Print and shaded views of the part. All mm, measured from the part's lowest x, y and z. Round coordinates to 2 decimals unless told otherwise and drop trailing zeros. Loops run counter-clockwise (first coordinate to the right, second up) from the corner with the lowest first, then second, coordinate; pieces in that order, holes last. Notation, with made-up numbers: (41.5, 31.5) -> (85.5, 31.5) arc R18 cw to (85.5, 47.5) -> close; hole circle Ø6 at (72.5, 72.25). An arc over 180 degrees is marked (long way). Answer as CSV lines item,"result".
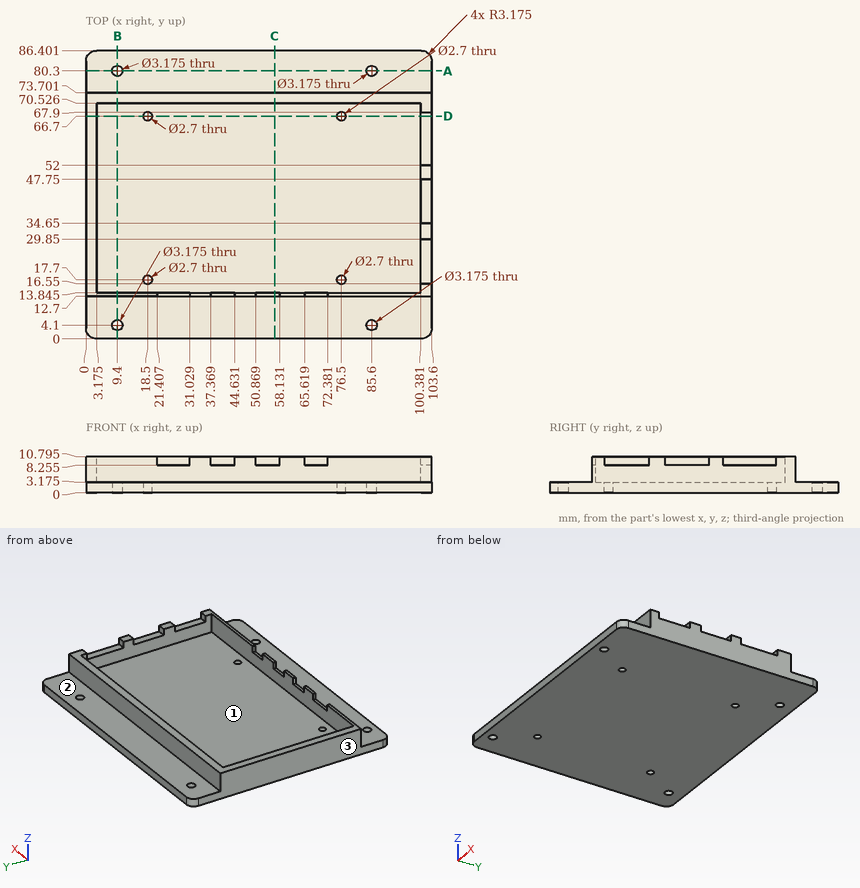
Q1. Slice it at B-B, the plane x = 9.4. Give the cut face in (y, z) (1 decimal), and give its area (3 significant figures).
Results:
outline,"(0, 0) -> (2.5, 0) -> (2.5, 3.2) -> (0, 3.2) -> close; (5.7, 0) -> (78.7, 0) -> (78.7, 3.2) -> (73.7, 3.2) -> (73.7, 10.8) -> (70.5, 10.8) -> (70.5, 3.2) -> (13.8, 3.2) -> (13.8, 10.8) -> (12.7, 10.8) -> (12.7, 3.2) -> (5.7, 3.2) -> close; (81.9, 0) -> (86.4, 0) -> (86.4, 3.2) -> (81.9, 3.2) -> close"
area,"287 mm2"
Q2. Slice it at D-D, the plane y = 66.7. Count the separate pieces of the cut face and the enclosed holes in it, and give its area (3 significant figures).
Results:
separate pieces,"3"
enclosed holes,"0"
area,"352 mm2"
Q3. Slice it at A-A, the plane y = 80.3. Give the cut face in (x, z) (1 decimal), and give its area (3 significant figures).
Results:
outline,"(0, 0) -> (7.8, 0) -> (7.8, 3.2) -> (0, 3.2) -> close; (11, 0) -> (84, 0) -> (84, 3.2) -> (11, 3.2) -> close; (87.2, 0) -> (103.6, 0) -> (103.6, 3.2) -> (87.2, 3.2) -> close"
area,"309 mm2"
Q4. Two-plate mould, pull along X, no slides. Class the marked faces 1, 2 and 3: pulls with the +X half, pulls with the -X half, needs draft (parallel to the pull), parting line crosses it, or undercut.
Results:
face 1,"undercut"
face 2,"needs draft"
face 3,"pulls with the -X half"
Q5. Slice it at C-C, the plane x = 56.5. Give the cut face in (y, z) (1 decimal), and give its area (3 significant figures).
Results:
outline,"(0, 0) -> (86.4, 0) -> (86.4, 3.2) -> (73.7, 3.2) -> (73.7, 10.8) -> (70.5, 10.8) -> (70.5, 3.2) -> (13.8, 3.2) -> (13.8, 8.3) -> (12.7, 8.3) -> (12.7, 3.2) -> (0, 3.2) -> close"
area,"304 mm2"
Q6. Drop flat-ended pins along their axis: pin 1 Ø1 at (x, z) = (45.5, 7.5) entering from -Y; pin 2 Ø0.8 at (x, z) = (101.5, 9.5) entering from +Y; pin 3 Ø1.3 at (x, y) = (55.5, 13.5) entering from +Z (3 decimals); pin 4 Ø3 at (x, y) = (9.4, 4.1) entering from +Z. Give the stop position or say it passes through.
Results:
pin 1,"y = 12.7"
pin 2,"y = 73.7"
pin 3,"z = 8.255"
pin 4,"through"
Q7. Probe L1, parallel to Y at x = 18.5, z = 0.9; L2, parallel to X at y = 80.3, z = 1.8; L3, parallel to X at y = 34.5, z = 7.5 (1 decimal). List the from-to ranges inside material, lowest first. Write a range as [from, to].
Results:
L1,"[0, 16.35], [19.05, 65.35], [68.05, 86.4]"
L2,"[0, 7.81], [10.99, 84.01], [87.19, 103.6]"
L3,"[0, 3.2], [100.4, 103.6]"
